Work out the finished part from the listing and answer in its coordinate system (mm). A direction names the side the tool comes from. Round coordinates to 2 decimals unless told otherwise and drop trailing zeros. Loops run counter-clockwise (first coordinate to the right, second up) from the corner with the lowest first, then second, coordinate; pieces in that order, holes last.
```python
from build123d import *

# Parameters (mm, degrees)
PRISM_DEPTH       = 3.1
CYLINDER021_R     = 2
CYLINDER021_DEPTH = 10
CYLINDER020_R     = 8
CYLINDER020_DEPTH = 5
CYLINDER023_R     = 6.1
CYLINDER023_DEPTH = 35
CYLINDER022_R     = 8
CYLINDER022_DEPTH = 35
FILLET_R          = 3


with BuildPart() as prism:
    # Prism → Prism (new body)
    with BuildSketch(Plane.XY.offset(1)):
        Polygon((3.25, 0), (1.625, 2.814583), (-1.625, 2.814583), (-3.25, 0), (-1.625, -2.814583), (1.625, -2.814583), align=None)
    extrude(amount=PRISM_DEPTH)


with BuildPart() as cylinder021:
    # Cylinder021 → Cylinder021 (new body)
    with BuildSketch(Plane.XY):
        Circle(CYLINDER021_R)
    extrude(amount=CYLINDER021_DEPTH)


with BuildPart() as cut017:
    # Cylinder020 → Cylinder020 (new body)
    with BuildSketch(Plane.XY):
        Circle(CYLINDER020_R)
    extrude(amount=CYLINDER020_DEPTH)

    # Cut015: cut Cylinder021
    add(cylinder021.part, mode=Mode.SUBTRACT)

    # Cut017: cut Prism
    add(prism.part, mode=Mode.SUBTRACT)


with BuildPart() as cylinder023:
    # Cylinder023 → Cylinder023 (new body)
    with BuildSketch(Plane.XY):
        Circle(CYLINDER023_R)
    extrude(amount=CYLINDER023_DEPTH)


with BuildPart() as fillet_body:
    # Cylinder022 → Cylinder022 (new body)
    with BuildSketch(Plane.XY):
        Circle(CYLINDER022_R)
    extrude(amount=CYLINDER022_DEPTH)

    # Cut016: cut Cylinder023
    add(cylinder023.part, mode=Mode.SUBTRACT)


with BuildPart() as fillet_body_1:
    # Cut016 placement: moved
    add(fillet_body.part.moved(Location((0, 0, 5))))

    # Fusion010: union Cut017
    add(cut017.part)

    # Fillet
    fillet_edges = [fillet_body_1.edges().sort_by_distance(p)[0] for p in [
        (-6.1, 0, 5),
    ]]
    fillet(fillet_edges, radius=FILLET_R)


solid = fillet_body_1.part
```
1. Consider probe 1 along Y at (x, z) = (0, 4.4); probe 2 along Y at (x, z) = (0, 25.5); probe 3 along X at (y, z) = (-0.25, 21.5). Determine where each line is inside the solid, lowest interval first.
Answer key:
probe 1: y = -8 to -2, 2 to 8
probe 2: y = -8 to -6.1, 6.1 to 8
probe 3: x = -8 to -6.09, 6.09 to 8
2. Find section B-B (z = 30). Write down the section's boundary in (x, y).
Answer key:
outline: circle Ø16 at (0, 0); hole circle Ø12.2 at (0, 0)
3. Determine the mould class of faces 1 (the face through (2.449, 1.388, 2.528)), 2 (the face through (2, -2, 0)), 3 (the face through (-0.434, -1.952, 0.493)), 4 (the face through (-1.73, -7.81, 19.72)) for opening direction Y: +Y half, -Y half, draft (parallel to the pull), parting line (faces both ways), or undercut.
Answer key:
face 1: undercut
face 2: draft
face 3: undercut
face 4: parting line
4. Find section C-C (x = 7.25). Write down the section's boundary in (y, z).
Answer key:
outline: (-3.38, 0) - (3.38, 0) - (3.38, 40) - (-3.38, 40) - close
5. Given pin 1 (1.5 mm diameter, centred on y = 1, z = 13, fed in from +X); pin 2 (1.5 mm diameter, centred on x = -0.5, z = 2.5, fed in from +Y); pin 3 (1.5 mm diameter, centred on x = 5, z = 25.5, fed in from +Y); pin 4 (6.5 mm diameter, centred on x = 0, y = 0, fed in from +Z), each flat-ended and moving along its own axis, determine where each tip first touches the part or whether it passes through.
Answer key:
pin 1: stops at x = 8
pin 2: stops at y = 8
pin 3: stops at y = 6.78
pin 4: stops at z = 5
6. Find section A-A (x = 0). Write down the section's boundary in (y, z).
Answer key:
outline: (-8, 0) - (-2, 0) - (-2, 1) - (-2.81, 1) - (-2.81, 4.1) - (-2, 4.1) - (-2, 5) - (-3.1, 5) arc R3 cw to (-6.1, 8) - (-6.1, 40) - (-8, 40) - close; (2, 0) - (8, 0) - (8, 40) - (6.1, 40) - (6.1, 8) arc R3 cw to (3.1, 5) - (2, 5) - (2, 4.1) - (2.81, 4.1) - (2.81, 1) - (2, 1) - close
7. Which of the six approach directions +Z, -Z, +X, -X, +Y, -Y give full straight-line access (tool end or side, diameter ignored) to faces 5 (the face through (2, -1, 5)), 6 (the face through (-2.426, 1.427, 2.528)), 7 (the face through (-2, -6, 40))?
Answer key:
face 5: +Z
face 6: none
face 7: +Z, +X, -X, +Y, -Y
